Here's how the part is built. I have some questions about the finished solid (model axes, mm). A direction names the side the tool comes from. Round coordinates to 2 decimals unless told otherwise and drop trailing zeros. Loops run counter-clockwise (first coordinate to the right, second up) from the corner with the lowest first, then second, coordinate; pieces in that order, holes last. Notation, with made-up numbers: (87.25, 24) - (119.25, 24) arc R18 ccw to (119.25, 58) - close; hole circle Ø3 at (77.25, 83.25). An arc over 180 degrees is marked (long way). Answer as a JSON object with one key per item and string values. Group by question number.
1) Which directions (+Z, -Z, +X, -X, +Y, -Y) give clear straight access to the entire face, cutting with the end or side of a thin tool? Please do faces 4 (the face through (-59.94, 2.64, 7.4)), 5 (the face through (-1, -19, 11)).
2) I want a section at D-D, the plane y = -29.5. Please give me the cut outline in (x, z).
3) I want a section at A-A, the plane x = 0. Please give me the cut outline in (y, z).
4) I want a section at B-B, the plane y = 0. Please give me the cut outline in (x, z).
5) If we mould it in two halves opening along X, with no side actions, what happens to faces 1 (the face through (41.5, 0, 11)), 2 (the face through (52.654, -21.831, 17.535)), 3 (the face through (-1, 14, 0))? For each: pulls with the +X half, pulls with the -X half, needs draft (parallel to the pull), parting line crosses it, or undercut.
6) I want a section at C-C, the plane z = 17.75. Please give me the cut outline in (x, y), then the cut area to 3 significant figures.
7) If I drill on line 1 along Y through (x, z) = (-1.5, 2.5); line 2 along Z through (x, y) = (-54, 26); line 3 along Y through (x, z) = (-13.5, 2.5), over which ranges is the centre line in solid material (lowest first)? Write a range as [from, to].
8) Will these pins go through, and if not, where does the flat tip stop? P1, Ø2, axis at y = 5.5, z = 1.5, coming from the +X side; P2, Ø9, axis at y = 8, z = 15.5, coming from the +X side; P3, Ø1.6, axis at x = 7.5, z = 1.5, coming from the -Y side.
from build123d import *

# Parameters (mm, degrees)
F0_R           = 60
F0_R_2         = 57
F2_DEPTH       = 15
F1_R           = 57
F1_R_2         = 54
F3_DEPTH       = 20
F4_R           = 57
F5_DEPTH       = 10
F7_R           = 54
F8_DEPTH       = 40
F9_W           = 15
F9_H           = 10
F10_DEPTH      = 279.5
F11_DEPTH      = 71.5
F13_R          = 60
F14_DEPTH      = 20
F15_W          = 72
F15_H          = 25
F16_DEPTH      = 20
F17_W          = 83
F17_H          = 38
F18_DEPTH      = 13
F18_DEPTH_BACK = 5
F19_R          = 60
F19_R_2        = 57
F20_DEPTH      = 5


# Not quite as in the source:
# - a feature names something its author has since deleted; it is built from what else it names


with BuildPart() as f2:
    # F0 (on Top) → F2 (new body)
    with BuildSketch(Plane.XY):
        Circle(F0_R)
        Circle(F0_R_2, mode=Mode.SUBTRACT)
    extrude(amount=F2_DEPTH)

    # F1 (on Top) → F3 (join)
    with BuildSketch(Plane.XY):
        Circle(F1_R)
        Circle(F1_R_2, mode=Mode.SUBTRACT)
    extrude(amount=F3_DEPTH)

    # F4 (on Top) → F5 (join)
    with BuildSketch(Plane.XY):
        Circle(F4_R)
    extrude(amount=F5_DEPTH)

    # F7 (on offset) → F8 (cut)
    with BuildSketch(Plane.XY.offset(45)):
        Circle(F7_R)
    extrude(amount=-F8_DEPTH, mode=Mode.SUBTRACT)

    # F9 (on Right) → F10 (cut)
    with BuildSketch(Plane.YZ):
        with Locations((32.5, 60)):
            Rectangle(F9_W, F9_H)
    extrude(amount=F10_DEPTH, mode=Mode.SUBTRACT)

    # F1 (on Top) → F11 (cut)
    with BuildSketch(Plane.XY):
        Circle(F1_R_2)
    extrude(amount=F11_DEPTH, mode=Mode.SUBTRACT)

    # F13 (on Top) → F14 (join)
    with BuildSketch(Plane.XY):
        Circle(F13_R)
    extrude(amount=F14_DEPTH)

    # F15 (on Top) → F16 (cut)
    with BuildSketch(Plane.XY):
        Rectangle(F15_W, F15_H)
    extrude(amount=F16_DEPTH, mode=Mode.SUBTRACT)

    # F17 (on offset) → F18 (cut, two sides)
    with BuildSketch(Plane.XY.offset(15)) as f18_sk:
        Rectangle(F17_W, F17_H)
    extrude(amount=-F18_DEPTH, mode=Mode.SUBTRACT)
    extrude(f18_sk.sketch, amount=F18_DEPTH_BACK, mode=Mode.SUBTRACT)

    # F19 (on face) → F20 (cut)
    with BuildSketch(Plane.XY.offset(20)):
        Circle(F19_R)
        Circle(F19_R_2, mode=Mode.SUBTRACT)
    extrude(amount=-F20_DEPTH, mode=Mode.SUBTRACT)


solid = f2.part
Outcome:
{
 "1": {"face 4": "+Z, -Z", "face 5": "+Z"},
 "2": {"outline": "(-52.25, 0) - (52.25, 0) - (52.25, 15) - (48.77, 15) - (48.77, 20) - (-48.77, 20) - (-48.77, 15) - (-52.25, 15) - close"},
 "3": {"outline": "(-60, 0) - (-12.5, 0) - (-12.5, 2) - (-19, 2) - (-19, 20) - (-57, 20) - (-57, 15) - (-60, 15) - close; (12.5, 0) - (60, 0) - (60, 15) - (57, 15) - (57, 20) - (19, 20) - (19, 2) - (12.5, 2) - close"},
 "4": {"outline": "(-60, 0) - (-36, 0) - (-36, 2) - (-41.5, 2) - (-41.5, 20) - (-57, 20) - (-57, 15) - (-60, 15) - close; (36, 0) - (60, 0) - (60, 15) - (57, 15) - (57, 20) - (41.5, 20) - (41.5, 2) - (36, 2) - close"},
 "5": {"face 1": "undercut", "face 2": "parting line crosses it", "face 3": "needs draft"},
 "6": {"outline": "circle Ø114 at (0, 0); hole (-41.5, -19) - (41.5, -19) - (41.5, 19) - (-41.5, 19) - close", "area": "7,050 mm^2"},
 "7": {"line 1": "[-59.98, -19], [19, 59.98]", "line 2": "[0, 15]", "line 3": "[-58.46, -19], [19, 58.46]"},
 "8": {"P1": "x = 59.83", "P2": "x = 59.9", "P3": "y = -59.62"}
}
